Design review of the part built by this model. Coordinates are the model's own, in mm. Face numbers are marked on the shaded views. A direction names the side the tool comes from. Coordinates: 2 decimals unless noted, no trailing zeros. Write each loop counter-clockwise with the first axis right and the second up, starting at its lowest first coordinate (ties: lowest second). Pieces come first, ordered by that corner, then holes. Notation, with made-up numbers: (-37.75, 74.25) - (-6.75, 74.25) arc R6 cw to (-6.75, 81.25) - close; hole circle Ø3 at (85, -16.5). An arc over 180 degrees is marked (long way). Use a Markdown table: item, result.
from build123d import *

# Parameters (mm, degrees)
SKETCH1_R               = 11
BOSS_EXTRUDE1_DEPTH     = 18
SKETCH2_R               = 20
BOSS_EXTRUDE2_DEPTH     = 10
SKETCH3_R               = 5
CUT_EXTRUDE1_DEPTH      = 1
CUT_EXTRUDE1_DEPTH_BACK = 19
SKETCH4_R               = 2.25
CUT_EXTRUDE2_DEPTH      = 7
CIRPATTERN1_COUNT       = 4
SKETCH5_R               = 2.25
CUT_EXTRUDE3_DEPTH      = 21
CIRPATTERN2_COUNT       = 2
CIRPATTERN2_ANGLE       = 90


with BuildPart() as part:
    # Sketch1 → Boss-Extrude1 (new body)
    with BuildSketch(Plane(origin=(0, 0, 0), x_dir=(1, 0, 0), z_dir=(0, 1, 0))):
        Circle(SKETCH1_R)
    extrude(amount=BOSS_EXTRUDE1_DEPTH)

    # Sketch2 → Boss-Extrude2 (add)
    with BuildSketch(Plane.XZ):
        Circle(SKETCH2_R)
    extrude(amount=-BOSS_EXTRUDE2_DEPTH)

    # Sketch3 → Cut-Extrude1 (cut, two sides)
    with BuildSketch(Plane(origin=(0, 18, 0), x_dir=(1, 0, 0), z_dir=(0, 1, 0))) as cut_extrude1_sk:
        Circle(SKETCH3_R)
    extrude(amount=CUT_EXTRUDE1_DEPTH, mode=Mode.SUBTRACT)
    extrude(cut_extrude1_sk.sketch, amount=-CUT_EXTRUDE1_DEPTH_BACK, mode=Mode.SUBTRACT)

    # Sketch4 → Cut-Extrude2 (cut)
    with BuildSketch(Plane.XZ):
        with Locations((-10.606601718, 10.606601718)):
            Circle(SKETCH4_R)
    cut_extrude2 = extrude(amount=-CUT_EXTRUDE2_DEPTH, mode=Mode.SUBTRACT)

    # CirPattern1: Cut-Extrude2 ×4 about axis
    cirpattern1_axis = Axis((0, 0, 0), (0, 1, 0))
    for i in range(1, CIRPATTERN1_COUNT):
        add(cut_extrude2.rotate(cirpattern1_axis, i * 360 / CIRPATTERN1_COUNT), mode=Mode.SUBTRACT)

    # Sketch5 → Cut-Extrude3 (cut, through all)
    with BuildSketch(Plane.XY):
        with Locations((0, 14)):
            Circle(SKETCH5_R)
        with Locations((0, 5)):
            Circle(SKETCH5_R)
    cut_extrude3 = extrude(amount=-CUT_EXTRUDE3_DEPTH, mode=Mode.SUBTRACT)

    # CirPattern2: Cut-Extrude3 ×2 about axis
    cirpattern2_axis = Axis((0, 18, 0), (0, 1, 0))
    for i in range(1, CIRPATTERN2_COUNT):
        add(cut_extrude3.rotate(cirpattern2_axis, i * CIRPATTERN2_ANGLE / (CIRPATTERN2_COUNT - 1)), mode=Mode.SUBTRACT)


solid = part.part
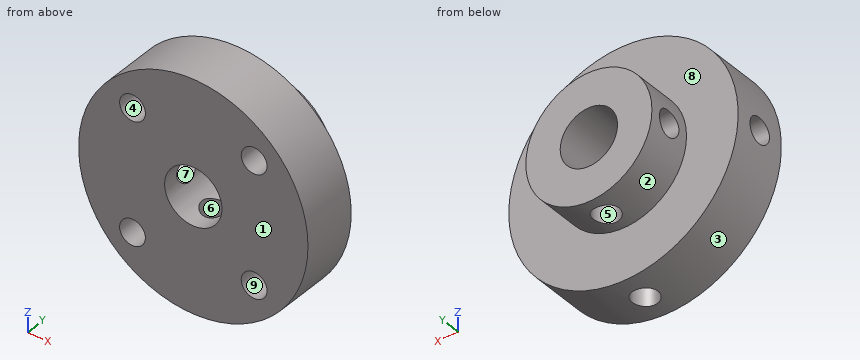
(1) Take a section at A-A on z = 0. Write out the cut boundary in (x, y), and give its area (4 significant figures).
Determined:
| item | result |
|---|---|
| outline | (-20, 0) - (-5, 0) - (-5, 2.75) - (-20, 2.75) - close; (-20, 7.25) - (-5, 7.25) - (-5, 11.75) - (-11, 11.75) - (-11, 10) - (-20, 10) - close; (-11, 16.25) - (-5, 16.25) - (-5, 18) - (-11, 18) - close; (5, 0) - (20, 0) - (20, 10) - (11, 10) - (11, 18) - (5, 18) - close |
| area | 301.5 mm2 |
(2) Machinability: for the marked faces 1, 2, 3, 4 and 5, which of the approach directions +Z, -Z, +X, -X, +Y, -Y give a long, thin tool a straight path to every point of the face, cutting with its end or side? Answer none if there is none.
Determined:
| item | result |
|---|---|
| face 1 | +Z, -Z, +X, -X, -Y |
| face 2 | +Y |
| face 3 | +Y, -Y |
| face 4 | -Y |
| face 5 | -Z |
(3) Take a section at C-C on y = 14.5. Write out the cut boundary in (x, z).
Determined:
| item | result |
|---|---|
| outline | (-10.78, -2.19) arc R11 ccw to (-2.19, -10.78) - (-2.19, -4.49) arc R5 cw to (-4.49, -2.19) - close; (-10.78, 2.19) - (-4.49, 2.19) arc R5 cw (long way) to (2.19, -4.49) - (2.19, -10.78) arc R11 ccw (long way) to start |
(4) Draft analysis for pull direction Y (two halves, no side actions). For the marked faces 6, 7, 8 and 9, state which applies: +Y half, -Y half, draft (parallel to the pull), parting line (faces both ways), or undercut.
Determined:
| item | result |
|---|---|
| face 6 | undercut |
| face 7 | undercut |
| face 8 | +Y half |
| face 9 | draft |
(5) Take a section at B-B on x = 0. Write out the cut boundary in (y, z).
Determined:
| item | result |
|---|---|
| outline | (0, -20) - (2.75, -20) - (2.75, -5) - (0, -5) - close; (0, 5) - (18, 5) - (18, 11) - (10, 11) - (10, 20) - (0, 20) - close; (7.25, -20) - (10, -20) - (10, -11) - (11.75, -11) - (11.75, -5) - (7.25, -5) - close; (16.25, -11) - (18, -11) - (18, -5) - (16.25, -5) - close |
(6) For pin 1 (2 mm diameter, centred on x = -11, z = -11, fed in from -Y); pin 2 (8 mm diameter, centred on x = 15.5, y = 11, fed in from +Z); pin 3 (8 mm diameter, centred on x = -10, y = 6.5, fed in from +Z); pin 4 (6 mm diameter, centred on y = 5, z = 0, fed in from -X), all flat-tipped, find the tip position at first contact; note any pin that passes through.
Determined:
| item | result |
|---|---|
| pin 1 | y = 7 |
| pin 2 | z = 16.27 |
| pin 3 | z = 19.08 |
| pin 4 | x = -20 |
(7) For L1, parallel to Y at x = 0, z = -6.75; L2, parallel to Y at x = -15, z = -5; L3, parallel to X at y = 2.75, z = 1, list the stretches that pass through material, from the lowest coordinate up. Write a range as from..to.
Determined:
| item | result |
|---|---|
| L1 | 0..2.75, 7.25..11.75, 16.25..18 |
| L2 | 0..10 |
| L3 | -19.97..-4.9, 4.9..19.97 |
(8) Take a section at D-D on z = -11.5. Write out the cut boundary in (x, y).
Determined:
| item | result |
|---|---|
| outline | (-16.36, 0) - (-12.67, 0) - (-12.67, 7) - (-8.54, 7) - (-8.54, 0) - (8.54, 0) - (8.54, 7) - (12.67, 7) - (12.67, 0) - (16.36, 0) - (16.36, 10) - (-16.36, 10) - close; hole circle Ø4.5 at (0, 5) |
